Verification items for the finished model (mm, model axes). Round coordinates to 2 decimals unless told otherwise and drop trailing zeros. Order: outer loops, then holes, each group sorted by start corner. A loop starts at its lowest first (then second) coordinate and runs counter-clockwise, first axis right, second up. Notation, with made-up numbers: (-16, 7) -> (32, 7) arc R25 ccw to (32, 28) -> close; hole circle Ø4 at (24, 21). An arc over 180 degrees is marked (long way). Answer in a Markdown table with one row per item. Add a question column.
Autodesk Inventor part; units mm, degrees
ref_plane "YZ Plane" through (0, 0, 0) normal (1, 0, 0) x (0, 1, 0)
ref_plane "XZ Plane" through (0, 0, 0) normal (0, 1, 0) x (-1, 0, 0)
ref_plane "XY Plane" through (0, 0, 0) normal (0, 0, 1) x (1, 0, 0)
sketch "Sketch1" plane through (0, 0, 0) normal (0, 0, 1) x (1, 0, 0)
  line L0 (0, 0) -> (25.4, 0)
  line L1 (25.4, 0) -> (25.4, 25.4)
  line L2 (25.4, 25.4) -> (0, 25.4)
  line L3 (0, 25.4) -> (0, 0)
  dimension "d0" = 25.4
  dimension "d1" = 25.4
extrude "Extrusion1" add sketch "Sketch1" along normal blind 279.4
shell "Shell1" thickness 1.143 removed faces 2 at (8.4667, 16.9333, 0) at (8.4667, 16.9333, 279.4)
sketch "Sketch2" plane through (25.4, 0, 0) normal (1, 0, 0) x (0, 0, -1)
  circle A0 centre (-259.5499, 12.7) radius 8.5725
  line L0 (-279.4, 0) -> (-279.4, 25.4)
  line L1 (0, 25.4) -> (-279.4, 25.4)
  circle A1 centre (-19.8501, 12.7) radius 8.5725
  line L2 (0, 0) -> (0, 25.4)
  dimension "d5" = 17.145
  dimension "d6" = 19.8501
  dimension "d7" = 12.7
  dimension "d8" = 17.145
  dimension "d9" = 19.8501
  dimension "d10" = 12.7
extrude "Extrusion2" cut sketch "Sketch2" against normal blind 279.4
sketch "Sketch3" plane through (0, 25.4, 0) normal (0, 1, 0) x (1, 0, 0)
  circle A0 centre (12.7, -12.7) radius 1.905
  line L0 (25.4, 0) -> (0, 0)
  line L1 (0, 0) -> (0, -279.4)
  circle A1 centre (12.7, -38.1) radius 1.905
  circle A2 centre (12.7, -63.5) radius 1.905
  circle A3 centre (12.7, -88.9) radius 1.905
  circle A4 centre (12.7, -114.3) radius 1.905
  circle A5 centre (12.7, -139.7) radius 1.905
  circle A6 centre (12.7, -165.1) radius 1.905
  circle A7 centre (12.7, -190.5) radius 1.905
  circle A8 centre (12.7, -215.9) radius 1.905
  circle A9 centre (12.7, -241.3) radius 1.905
  circle A10 centre (12.7, -266.7) radius 1.905
  dimension "d13" = 3.81
  dimension "d14" = 12.7
  dimension "d15" = 12.7
  dimension "d18" = 25.4
extrude "Extrusion3" cut sketch "Sketch3" against normal blind 279.4
sketch "Sketch4" plane through (25.4, 0, 0) normal (1, 0, 0) x (0, 0, -1)
  circle A0 centre (-255.4224, 12.7) radius 1.905
  line L0 (0, 25.4) -> (-279.4, 25.4)
  circle A1 centre (-259.5499, 12.7) radius 8.5725
  circle A2 centre (-230.0224, 12.7) radius 1.905
  circle A3 centre (-204.6224, 12.7) radius 1.905
  circle A4 centre (-179.2224, 12.7) radius 1.905
  circle A5 centre (-153.8224, 12.7) radius 1.905
  circle A6 centre (-128.4224, 12.7) radius 1.905
  circle A7 centre (-103.0224, 12.7) radius 1.905
  circle A8 centre (-77.6224, 12.7) radius 1.905
  circle A9 centre (-52.2224, 12.7) radius 1.905
  point P0 (0, 0)
  dimension "d25" = 3.81
  dimension "d26" = 12.7
  dimension "d27" = 4.1275
  dimension "d30" = 25.4
extrude "Extrusion4" cut sketch "Sketch4" against normal blind 279.4 contours A2 | A3 | A4 | A5 | A6 | A7 | A8 | A9
equation "\"d8\" = d5"
equation "\"d9\" = d6"
equation "\"d10\" = d7"
properties part number "Support Pivs 11"
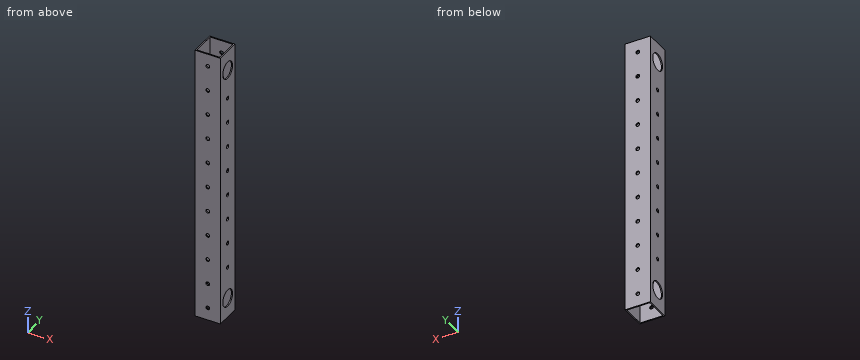
1) Cross-section at C-C, the plane y = 18.5. Record the boundary of the cut face in (x, z), and give its area (3 significant figures).
2) Cross-section at B-B, the plane z = 43. Record the boundary of the cut face in (x, y).
3) Thickness scan on L1, parallel to Y at x = 24, z = 233.5; L2, parallel to X at y = 24.8, z = 12.7 (3 decimals). Record the ranges inside material, lowest first. Write a range as [from, to].
4) Cross-section at A-A, the plane x = 21.75. Record the boundary of the cut face in (y, z).
Results below:
| question | item | result |
|---|---|---|
| 1 | outline | (0, 0) -> (1.14, 0) -> (1.14, 13.54) -> (0, 13.54) -> close; (0, 26.16) -> (1.14, 26.16) -> (1.14, 253.24) -> (0, 253.24) -> close; (0, 265.86) -> (1.14, 265.86) -> (1.14, 279.4) -> (0, 279.4) -> close; (24.26, 0) -> (25.4, 0) -> (25.4, 13.54) -> (24.26, 13.54) -> close; (24.26, 26.16) -> (25.4, 26.16) -> (25.4, 253.24) -> (24.26, 253.24) -> close; (24.26, 265.86) -> (25.4, 265.86) -> (25.4, 279.4) -> (24.26, 279.4) -> close |
| 1 | area | 581 mm² |
| 2 | outline | (0, 0) -> (25.4, 0) -> (25.4, 25.4) -> (0, 25.4) -> close; hole (1.14, 1.14) -> (24.26, 1.14) -> (24.26, 24.26) -> (1.14, 24.26) -> close |
| 3 | L1 | [0, 1.14], [24.26, 25.4] |
| 3 | L2 | [0, 10.795], [14.605, 25.4] |
| 4 | outline | (0, 0) -> (1.14, 0) -> (1.14, 279.4) -> (0, 279.4) -> close; (24.26, 0) -> (25.4, 0) -> (25.4, 279.4) -> (24.26, 279.4) -> close |
